from build123d import *

# Parameters (mm, degrees)
F0_R      = 2.35
F1_DEPTH  = 2.6
F2_R      = 2
F3_DEPTH  = 4
F4_R      = 1.6
F5_DEPTH  = 0.75
F6_R      = 0.75
F7_DEPTH  = 2.5
F8_R      = 1.15
F9_DEPTH  = 0.5
F10_R     = 0.75
F11_DEPTH = 2.5
F12_R     = 1.25
F13_DEPTH = 0.5


with BuildPart() as f1:
    # F0 (on Front) → F1 (new body)
    with BuildSketch(Plane.XZ):
        Circle(F0_R)
    extrude(amount=F1_DEPTH)

    # F2 (on face) → F3 (join)
    with BuildSketch(Plane.XZ.offset(2.6)):
        Circle(F2_R)
    extrude(amount=F3_DEPTH)

    # F4 (on face) → F5 (join)
    with BuildSketch(Plane(origin=(0, 0, 0), x_dir=(-1, 0, 0), z_dir=(0, 1, 0))):
        Circle(F4_R)
    extrude(amount=F5_DEPTH)

    # F6 (on face) → F7 (join)
    with BuildSketch(Plane(origin=(0, 0.75, 0), x_dir=(-1, 0, 0), z_dir=(0, 1, 0))):
        Circle(F6_R)
    extrude(amount=F7_DEPTH)

    # F8 (on face) → F9 (join)
    with BuildSketch(Plane(origin=(0, 3.25, 0), x_dir=(-1, 0, 0), z_dir=(0, 1, 0))):
        Circle(F8_R)
    extrude(amount=F9_DEPTH)

    # F10 (on face) → F11 (join)
    with BuildSketch(Plane(origin=(0, 3.75, 0), x_dir=(-1, 0, 0), z_dir=(0, 1, 0))):
        Circle(F10_R)
    extrude(amount=F11_DEPTH)

    # F12 (on face) → F13 (join)
    with BuildSketch(Plane(origin=(0, 6.25, 0), x_dir=(-1, 0, 0), z_dir=(0, 1, 0))):
        Circle(F12_R)
    extrude(amount=F13_DEPTH)


solid = f1.part
Design review of the part built by this model. Coordinates are the model's own, in mm. A direction names the side the tool comes from. Give positions to 0.01 mm unless a question says otherwise; leave off trailing zeros. Write each loop counter-clockwise with the first axis right and the second up, starting at its lowest first coordinate (ties: lowest second). Pieces come first, ordered by that corner, then holes. Notation, with made-up numbers: M 74,88 L 112,88 A17 ccw 112,113 Z; hole C -2.5,23 d2. An arc over 180 degrees is marked long. Answer as a JSON object with one key per item and string values. Group by question number.
1) We need section D-D (y = 1.25). Give the boundary of the cut face in (x, z).
2) We need section A-A (z = 0). Give the boundary of the cut face in (x, y), and give its area (3 significant figures).
3) Tool access review of faces 1 (the face through (0, 0, -2)), 2 (the face through (-0.509, -1.282, -2.294)), 3 (the face through (0.91, 3.5, -0.7)), 4 (the face through (0, -5, -2)): name each direction out of +Z, -Z, +X, -X, +Y, -Y from which nothing blocks a thin tool from reaching the whole face with its end or side.
4) We need section B-B (x = 0). Give the boundary of the cut face in (y, z), and give its area (3 significant figures).
5) We need section C-C (x = -0.9). Give the boundary of the cut face in (y, z).
6) Mouldability with a two-part tool opening along Y and no side actions: class faces 5 (the face through (0, 6.75, 0)), 6 (the face through (0.27, 6.5, -1.22)), 7 (the face through (0, 6.25, -1)) as released by +Y, released by -Y, zero draft, split by the parting line, or undercut.
7) For line 1 along Y through (x, z) = (-0.75, 0.8); line 2 along Y through (x, z) = (0.7, -1); line 3 along Y through (x, z) = (2.15, 0.25), list the stretches that pass through material, from the lowest coordinate up.
Answer key:
{
 "1": {"outline": "C 0,0 d1.5"},
 "2": {"outline": "M -2.35,-2.6 L -2,-2.6 L -2,-6.6 L 2,-6.6 L 2,-2.6 L 2.35,-2.6 L 2.35,0 L 1.6,0 L 1.6,0.75 L 0.75,0.75 L 0.75,3.25 L 1.15,3.25 L 1.15,3.75 L 0.75,3.75 L 0.75,6.25 L 1.25,6.25 L 1.25,6.75 L -1.25,6.75 L -1.25,6.25 L -0.75,6.25 L -0.75,3.75 L -1.15,3.75 L -1.15,3.25 L -0.75,3.25 L -0.75,0.75 L -1.6,0.75 L -1.6,0 L -2.35,0 Z", "area": "40.5 mm²"},
 "3": {"face 1": "+Y", "face 2": "+Y, -Y", "face 3": "none", "face 4": "-Y"},
 "4": {"outline": "M -6.6,-2 L -2.6,-2 L -2.6,-2.35 L 0,-2.35 L 0,-1.6 L 0.75,-1.6 L 0.75,-0.75 L 3.25,-0.75 L 3.25,-1.15 L 3.75,-1.15 L 3.75,-0.75 L 6.25,-0.75 L 6.25,-1.25 L 6.75,-1.25 L 6.75,1.25 L 6.25,1.25 L 6.25,0.75 L 3.75,0.75 L 3.75,1.15 L 3.25,1.15 L 3.25,0.75 L 0.75,0.75 L 0.75,1.6 L 0,1.6 L 0,2.35 L -2.6,2.35 L -2.6,2 L -6.6,2 Z", "area": "40.5 mm²"},
 "5": {"outline": "M -6.6,-1.79 L -2.6,-1.79 L -2.6,-2.17 L 0,-2.17 L 0,-1.32 L 0.75,-1.32 L 0.75,1.32 L 0,1.32 L 0,2.17 L -2.6,2.17 L -2.6,1.79 L -6.6,1.79 Z; M 3.25,-0.72 L 3.75,-0.72 L 3.75,0.72 L 3.25,0.72 Z; M 6.25,-0.87 L 6.75,-0.87 L 6.75,0.87 L 6.25,0.87 Z"},
 "6": {"face 5": "released by +Y", "face 6": "zero draft", "face 7": "undercut"},
 "7": {"line 1": "y = -6.6 to 0.75, 3.25 to 3.75, 6.25 to 6.75", "line 2": "y = -6.6 to 0.75, 6.25 to 6.75", "line 3": "y = -2.6 to 0"}
}
